Part print with two shaded views. Sizes in mm from the minimum x, y, z corner. A direction names the side the tool comes from. Give positions to 0.01 mm unless a question says otherwise; leave off trailing zeros. Order: outer loops, then holes, each group sorted by start corner. A loop starts at its lowest first (then second) coordinate and runs counter-clockwise, first axis right, second up. Notation, with made-up numbers: M -16,40.5 L 41,40.5 A5 cw 41,49.5 Z; hole C -10.75,4 d9. An arc over 180 degrees is marked long. Return JSON: item names as keys, results as strings.
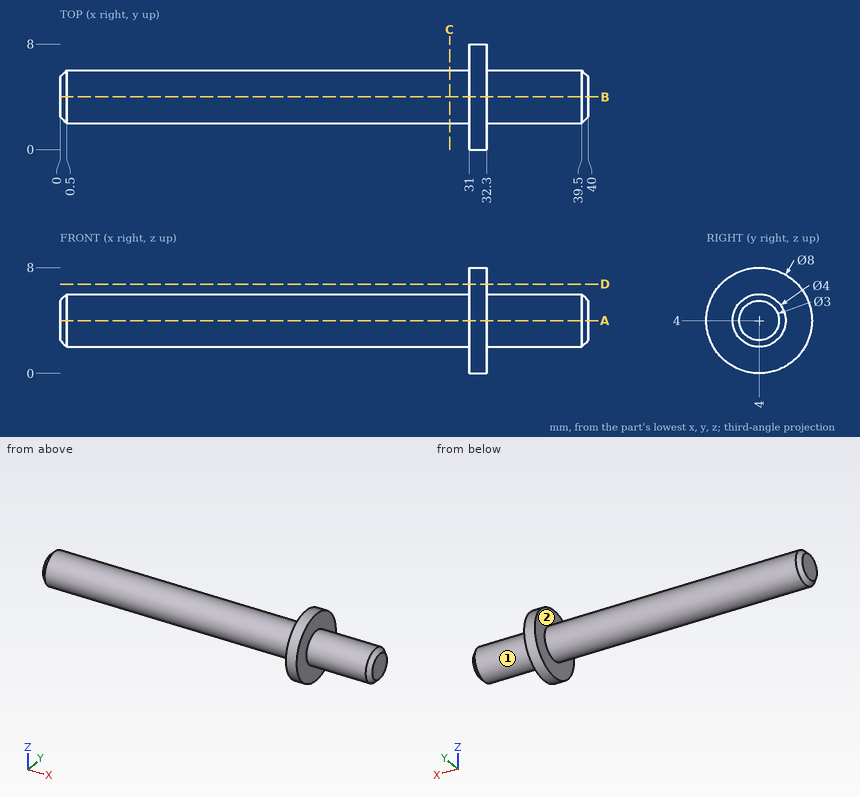
Q1. Probe line 1 along X through (y, z) = (1, 3); line 2 along Z through (x, y) = (25, 4); line 3 along Y through (x, z) = (3.5, 2.5). List the from-to ranges inside material, lowest first.
Established:
{"line 1": "x = 31 to 32.3", "line 2": "z = 2 to 6", "line 3": "y = 2.68 to 5.32"}
Q2. Band-saw the part on A-A (z = 4). Give the cut face in (x, y).
Established:
{"outline": "M 0,2.5 L 0.5,2 L 31,2 L 31,0 L 32.3,0 L 32.3,2 L 39.5,2 L 40,2.5 L 40,5.5 L 39.5,6 L 32.3,6 L 32.3,8 L 31,8 L 31,6 L 0.5,6 L 0,5.5 Z"}
Q3. 3-axis set-ups, long thin cutter, end or side, ignore diameter. For the marked faces 1 and 2: which of +Z, -Z, +X, -X, +Y, -Y reach the whole face in a straight line?
Established:
{"face 1": "+X", "face 2": "-X"}
Q4. Band-saw the part on C-C (x = 29.5). Give the cut face in (y, z), then the cut area to 3 significant figures.
Established:
{"outline": "C 4,4 d4", "area": "12.6 mm²"}
Q5. Band-saw the part on D-D (z = 6.75). Give the cut face in (x, y), then the cut area to 3 significant figures.
Established:
{"outline": "M 31,1.1 L 32.3,1.1 L 32.3,6.9 L 31,6.9 Z", "area": "7.55 mm²"}
Q6. Pin check, flat tips, straight feed: pin 1 (4 mm diameter, centred on x = 21, z = 5, fed in from -Y); pin 2 (1 mm diameter, centred on y = 6.5, z = 7, fed in from -X); pin 3 (2.5 mm diameter, centred on y = 4, z = 3, fed in from -X). Stop position of each tip, or through.
Established:
{"pin 1": "stops at y = 2", "pin 2": "stops at x = 31", "pin 3": "stops at x = 0"}
